from build123d import *

# Parameters (mm, degrees)
SKETCH2_W           = 91.809324831
SKETCH2_H           = 104
BOSS_EXTRUDE1_DEPTH = 2.54
SKETCH1_R           = 2
CUT_EXTRUDE1_DEPTH  = 536.483262079
CUT_EXTRUDE2_DEPTH  = 10
FILLET1_R           = 5


with BuildPart() as part:
    # Sketch2 → Boss-Extrude1 (new body)
    with BuildSketch(Plane.XY):
        with Locations((-386.858920313, 263.359404222)):
            Rectangle(SKETCH2_W, SKETCH2_H)
    extrude(amount=BOSS_EXTRUDE1_DEPTH)

    # Sketch1 → Cut-Extrude1 (cut, through all)
    with BuildSketch(Plane.XY):
        with Locations((-343.954257897, 311.359404222)):
            Circle(SKETCH1_R)
        with Locations((-429.763582728, 311.359404222)):
            Circle(SKETCH1_R)
        with Locations((-429.763582728, 215.359404222)):
            Circle(SKETCH1_R)
        with Locations((-343.954257897, 215.359404222)):
            Circle(SKETCH1_R)
    extrude(amount=CUT_EXTRUDE1_DEPTH, mode=Mode.SUBTRACT)

    # Sketch3 → Cut-Extrude2 (cut)
    with BuildSketch(Plane(origin=(0, 0, 0), x_dir=(-1, 0, 0), z_dir=(0, 0, -1))):
        with BuildLine():
            Line((380.954257897, 263.359404222), (340.954257897, 263.359404222))
            Line((340.954257897, 263.359404222), (340.954257897, 223.359404222))
            ThreePointArc((340.954257897, 223.359404222), (369.238529145, 235.075132974), (380.954257897, 263.359404222))
        make_face()
        with BuildLine():
            Line((340.954257897, 303.359404222), (340.954257897, 263.359404222))
            Line((340.954257897, 263.359404222), (380.954257897, 263.359404222))
            ThreePointArc((380.954257897, 263.359404222), (369.238529145, 291.643675469), (340.954257897, 303.359404222))
        make_face()
        with BuildLine():
            ThreePointArc((432.763582728, 303.359404222), (404.47931148, 291.643675469), (392.763582728, 263.359404222))
            Line((392.763582728, 263.359404222), (432.763582728, 263.359404222))
            Line((432.763582728, 263.359404222), (432.763582728, 303.359404222))
        make_face()
        with BuildLine():
            Line((432.763582728, 263.359404222), (392.763582728, 263.359404222))
            ThreePointArc((392.763582728, 263.359404222), (404.47931148, 235.075132974), (432.763582728, 223.359404222))
            Line((432.763582728, 223.359404222), (432.763582728, 263.359404222))
        make_face()
    extrude(amount=-CUT_EXTRUDE2_DEPTH, mode=Mode.SUBTRACT)

    # Fillet1
    fillet1_edges = [part.edges().sort_by_distance(p)[0] for p in [
        (-340.954257897, 303.359404222, 1.27),
        (-340.954257897, 223.359404222, 1.27),
        (-432.763582728, 303.359404222, 1.27),
        (-432.763582728, 223.359404222, 1.27),
        (-432.763582728, 211.359404222, 1.27),
        (-340.954257897, 211.359404222, 1.27),
        (-340.954257897, 315.359404222, 1.27),
        (-432.763582728, 315.359404222, 1.27),
    ]]
    fillet(fillet1_edges, radius=FILLET1_R)


solid = part.part
The model under review builds one solid part; all positions refer to its coordinate system, in mm. A direction names the side the tool comes from. Round coordinates to 2 decimals unless told otherwise and drop trailing zeros. Write each loop counter-clockwise with the first axis right and the second up, starting at its lowest first coordinate (ties: lowest second). Pieces come first, ordered by that corner, then holes. Notation, with made-up numbers: (16, 9.5) - (29, 9.5) arc R28 ccw to (29, 36.5) - close; hole circle Ø5 at (57, -5.75). An arc over 180 degrees is marked (long way). One line per item, written item: value. Start each with the question number.
1. Consider section A-A on x = -348.5. Write out the cut boundary in (y, z).
2. Consider section D-D on y = 233. Write out the cut boundary in (x, z).
3. Consider section B-B on z = 1.2. Write out the cut boundary in (x, y).
4. Machinability: for faces 1 (the face through (-342.19, 304.79, 1.29)), 2 (the face through (-387, 211.359, 1)), 3 (the face through (-431.524, 221.933, 1.288)), which of the approach directions +Z, -Z, +X, -X, +Y, -Y give a long, thin tool a straight path to every point of the face, cutting with its end or side? Answer none if there is none.
5. The part is to be moulded in two halves that separate along X. For faces 4 (the face through (-388, 264, 2.54)), 5 (the face through (-342.458, 313.934, 1.288)), 6 (the face through (-431.35, 214.14, 1.25)), 7 (the face through (-431.35, 310.14, 1.25)), say which applies: released by +X, released by -X, zero draft, split by the parting line, or undercut.
6. To check wall thickness, follow L1, parallel to X at y = 310.5, z = 1.85; L2, parallel to Y at x = -418, z = 0.85; L3, parallel to Y at x = -348.5, z = 0.2. State the ranges of each line that lie inside material, in increasing order. Write a range as from..to.
7. Consider section C-C on x = -377.5. Write out the cut boundary in (y, z).
8. Clearance check with flat-ended pins moving along their axes: P1, Ø3, axis at x = -429.76, y = 215.36, coming from the +Z side; P2, Ø1.5, axis at y = 293, z = 1, coming from the -X side. State where each tip first meets the part, or that it passes through.
Checks:
1. outline: (211.36, 0) - (224.08, 0) - (224.08, 2.54) - (211.36, 2.54) - close; (302.64, 0) - (315.36, 0) - (315.36, 2.54) - (302.64, 2.54) - close
2. outline: (-406.72, 0) - (-367, 0) - (-367, 2.54) - (-406.72, 2.54) - close
3. outline: (-432.76, 216.36) arc R5 ccw to (-427.76, 211.36) - (-345.95, 211.36) arc R5 ccw to (-340.95, 216.36) - (-340.95, 218.64) arc R5 ccw to (-345.4, 223.61) arc R40 cw to (-345.4, 303.11) arc R5 ccw to (-340.95, 308.08) - (-340.95, 310.36) arc R5 ccw to (-345.95, 315.36) - (-427.76, 315.36) arc R5 ccw to (-432.76, 310.36) - (-432.76, 308.08) arc R5 ccw to (-428.32, 303.11) arc R40 cw to (-428.32, 223.61) arc R5 ccw to (-432.76, 218.64) - close; hole circle Ø4 at (-429.76, 215.36); hole circle Ø4 at (-429.76, 311.36); hole circle Ø4 at (-343.95, 215.36); hole circle Ø4 at (-343.95, 311.36)
4. face 1: +Z, -Z, +X
4. face 2: +Z, -Z, +X, -X, -Y
4. face 3: +Z, -Z, -X
5. face 4: zero draft
5. face 5: released by +X
5. face 6: undercut
5. face 7: undercut
6. L1: x = -432.76..-431.57, -427.96..-345.76, -342.15..-340.96
6. L2: y = 211.36..226.18, 300.54..315.36
6. L3: y = 211.36..224.08, 302.64..315.36
7. outline: (211.36, 0) - (247.1, 0) - (247.1, 2.54) - (211.36, 2.54) - close; (279.62, 0) - (315.36, 0) - (315.36, 2.54) - (279.62, 2.54) - close
8. P1: passes through
8. P2: stops at x = -406.76
